Verification items for the finished model (mm, model axes). Round coordinates to 2 decimals unless told otherwise and drop trailing zeros. Order: outer loops, then holes, each group sorted by start corner. A loop starts at its lowest first (then second) coordinate and runs counter-clockwise, first axis right, second up. Notation, with made-up numbers: (79, 24.25) -> (91, 24.25) arc R20 cw to (91, 59.25) -> close; hole circle Ø4 at (11.25, 26.5). An arc over 180 degrees is marked (long way). Put each result on its own line as item: value.
```python
from build123d import *

# Parameters (mm, degrees)
SKETCH3_R           = 2.032
BOSS_EXTRUDE1_DEPTH = 28.575


with BuildPart() as part:
    # Sketch3 → Boss-Extrude1 (new body)
    with BuildSketch(Plane(origin=(0, 0, 0), x_dir=(1, 0, 0), z_dir=(0, 1, 0))):
        with BuildLine():
            Line((-27.78125, 0), (-27.78125, 25.4))
            Line((-27.78125, 25.4), (-11.361506121, 25.4))
            ThreePointArc((-11.361506121, 25.4), (-9.864796768, 24.341666667), (-10.363699885, 22.577777778))
            ThreePointArc((-10.363699885, 22.577777778), (-15.08125, 12.7), (-10.363699885, 2.822222222))
            ThreePointArc((-10.363699885, 2.822222222), (-9.864796768, 1.058333333), (-11.361506121, 0))
            Line((-11.361506121, 0), (-27.78125, 0))
        make_face()
        with Locations((-21.034375, 6.35)):
            Circle(SKETCH3_R, mode=Mode.SUBTRACT)
        with Locations((-21.034375, 19.05)):
            Circle(SKETCH3_R, mode=Mode.SUBTRACT)
    extrude(amount=BOSS_EXTRUDE1_DEPTH)


solid = part.part
```
Item 1: Depth check by flat-ended pin: pin 1 Ø2 at (y, z) = (8, -20) entering from +X; pin 2 Ø3 at (y, z) = (13, -15) entering from +X. Enter the tip coordinate at first touch or a pass-through.
Geometry check:
pin 1: x = -11.99
pin 2: x = -14.5
Item 2: Sectioned sample at B-B, the plane y = 15. Give the number of separate pieces and of enclosed holes in the cut face, then the cut area to 3 significant figures.
Geometry check:
separate pieces: 1
enclosed holes: 2
area: 353 mm2
Item 3: Sectioned sample at C-C, the plane z = -19.05. Record the boundary of the cut face in (x, y) (3 decimals), then the cut area to 3 significant figures.
Geometry check:
outline: (-27.781, 0) -> (-23.066, 0) -> (-23.066, 28.575) -> (-27.781, 28.575) -> close; (-19.002, 0) -> (-13.38, 0) -> (-13.38, 28.575) -> (-19.002, 28.575) -> close
area: 295 mm2
Item 4: Release check for a two-part mould opening along X. For faces 1 (the face through (-19, 14, 0)), 2 (the face through (-23.064, 14.087, -6.439)), 3 (the face through (-9.856, 14.087, -1.084)) record: pulls with the +X half, pulls with the -X half, needs draft (parallel to the pull), parting line crosses it, or undercut.
Geometry check:
face 1: needs draft
face 2: undercut
face 3: pulls with the +X half
Item 5: Sectioned sample at D-D, the plane x = -20.75. Record the boundary of the cut face in (y, z) (3 decimals).
Geometry check:
outline: (0, -25.4) -> (28.575, -25.4) -> (28.575, -21.062) -> (0, -21.062) -> close; (0, -17.038) -> (28.575, -17.038) -> (28.575, -8.362) -> (0, -8.362) -> close; (0, -4.338) -> (28.575, -4.338) -> (28.575, 0) -> (0, 0) -> close
Item 6: Material ranges on line 1 along Z through (x, y) = (-20.5, 25.25); line 2 along Z through (x, y) = (-19.5, 15.5); line 3 along X through (y, z) = (25, -5.75), recorded low to high.
Geometry check:
line 1: -25.4 to -21.01, -17.09 to -8.31, -4.39 to 0
line 2: -25.4 to -20.38, -17.72 to -7.68, -5.02 to 0
line 3: -27.78 to -22.98, -19.09 to -13.01
Item 7: Sectioned sample at A-A, the plane x = -13.25. Record the boundary of the cut face in (y, z) (3 decimals).
Geometry check:
outline: (0, -25.4) -> (28.575, -25.4) -> (28.575, -19.27) -> (0, -19.27) -> close; (0, -6.13) -> (28.575, -6.13) -> (28.575, 0) -> (0, 0) -> close
